Could you check a few things on this drawing? It's one solid part, dimensions in mm from its lowest x, y, z. A direction names the side the tool comes from. Round coordinates to 2 decimals unless told otherwise and drop trailing zeros. Loops run counter-clockwise (first coordinate to the right, second up) from the corner with the lowest first, then second, coordinate; pieces in that order, holes last. Notation, with made-up numbers: M 29,19 L 81,19 A11 ccw 81,34 Z; hole C 74,-38.5 d3. An arc over 180 degrees is marked long. Answer as a JSON object with one key per item and string values.
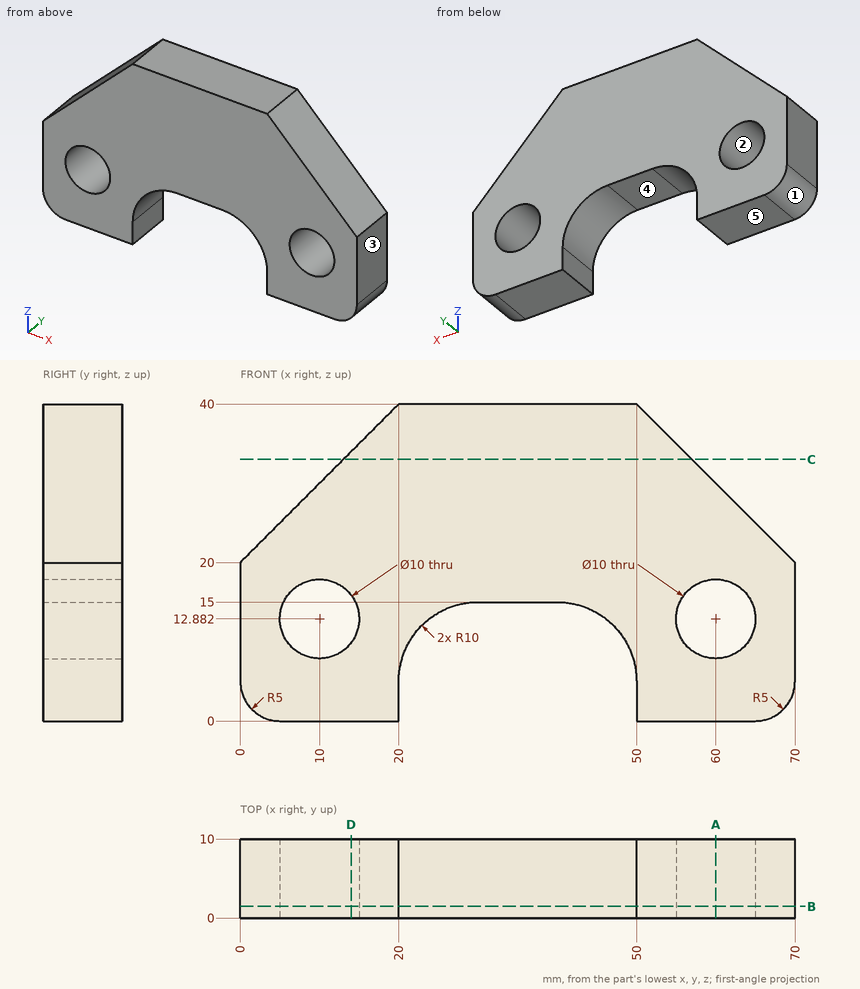
Item 1: If we mould it in two halves opening along Z, with no side actions, what happens to the marked faces 1, 2 and 3? For each: pulls with the +Z half, pulls with the -Z half, needs draft (parallel to the pull), parting line crosses it, or undercut.
Resolved:
{"face 1": "pulls with the -Z half", "face 2": "undercut", "face 3": "needs draft"}
Item 2: Please list where these lines run through material, in increasing order: probe 1 along Z at (x, y) = (60, 7); probe 2 along X at (y, z) = (8.25, 13.5); probe 3 along X at (y, z) = (7, 16). Write a range as from..to.
Resolved:
{"probe 1": "0..7.88, 17.88..30", "probe 2": "0..5.04, 14.96..24.73, 45.27..55.04, 64.96..70", "probe 3": "0..6.09, 13.91..56.09, 63.91..70"}
Item 3: On a 3-axis mill with a long thin cutter (end or side, diameter ignored), from which of +Z, -Z, +X, -X, +Y, -Y can I reach the whole of each face in a straight line? I mean the marked faces 4 and 5. Say none if no direction works.
Resolved:
{"face 4": "-Z, +Y, -Y", "face 5": "-Z, +X, -X, +Y, -Y"}
Item 4: I want a section at D-D, the plane x = 14. Please give me the cut outline in (y, z).
Resolved:
{"outline": "M 0,0 L 10,0 L 10,9.88 L 0,9.88 Z; M 0,15.88 L 10,15.88 L 10,34 L 0,34 Z"}
Item 5: I want a section at C-C, the plane z = 33. Please give me the cut outline in (x, y).
Resolved:
{"outline": "M 13,0 L 57,0 L 57,10 L 13,10 Z"}
Item 6: I'm going to push flat-ended pins straight in: pin 1 Ø2.5 at (y, z) = (4.5, 2) entering from -X; pin 2 Ø1.5 at (y, z) = (7, 1.5) entering from +X (1 decimal); pin 3 Ø1 at (y, z) = (7.5, 23) entering from -X. Where does each tip first touch, or does it pass through?
Resolved:
{"pin 1": "x = 0.32", "pin 2": "x = 69.2", "pin 3": "x = 2.5"}
Item 7: I want a section at B-B, the plane y = 1.5. Please give me the cut outline in (x, z).
Resolved:
{"outline": "M 0,5 A5 ccw 5,0 L 20,0 L 20,5 A10 cw 30,15 L 40,15 A10 cw 50,5 L 50,0 L 65,0 A5 ccw 70,5 L 70,20 L 50,40 L 20,40 L 0,20 Z; hole C 10,12.88 d10; hole C 60,12.88 d10"}
Item 8: I want a section at A-A, the plane x = 60. Please give me the cut outline in (y, z), then the cut area to 3 significant figures.
Resolved:
{"outline": "M 0,0 L 10,0 L 10,7.88 L 0,7.88 Z; M 0,17.88 L 10,17.88 L 10,30 L 0,30 Z", "area": "200 mm²"}
